```python
from build123d import *

# Parameters (mm, degrees)
F0_R     = 40
F1_DEPTH = 2.74
F2_R     = 8
F3_DEPTH = 40
F4_R     = 3.5
F5_DEPTH = 9.9
F7_DEPTH = 155.2


with BuildPart() as f1:
    # F0 (on Top) → F1 (new body)
    with BuildSketch(Plane.XY):
        Circle(F0_R)
    extrude(amount=F1_DEPTH)

    # F2 (on face) → F3 (join)
    with BuildSketch(Plane(origin=(0, 0, 0), x_dir=(1, 0, 0), z_dir=(0, 0, -1))):
        Circle(F2_R)
    extrude(amount=-F3_DEPTH)

    # F4 (on face) → F5 (join)
    with BuildSketch(Plane(origin=(0, 0, 0), x_dir=(1, 0, 0), z_dir=(0, 0, -1))):
        with BuildLine():
            Line((-38.7, -44.7), (38.7, -44.7))
            ThreePointArc((38.7, -44.7), (42.942641, -42.942641), (44.7, -38.7))
            Line((44.7, -38.7), (44.7, 38.7))
            ThreePointArc((44.7, 38.7), (42.942641, 42.942641), (38.7, 44.7))
            Line((38.7, 44.7), (-38.7, 44.7))
            ThreePointArc((-38.7, 44.7), (-42.942641, 42.942641), (-44.7, 38.7))
            Line((-44.7, 38.7), (-44.7, -38.7))
            ThreePointArc((-44.7, -38.7), (-42.942641, -42.942641), (-38.7, -44.7))
        make_face()
        with Locations((-35.355339, -35.355339)):
            Circle(F4_R, mode=Mode.SUBTRACT)
        with Locations((35.355339, -35.355339)):
            Circle(F4_R, mode=Mode.SUBTRACT)
        with Locations((-35.355339, 35.355339)):
            Circle(F4_R, mode=Mode.SUBTRACT)
        with Locations((35.355339, 35.355339)):
            Circle(F4_R, mode=Mode.SUBTRACT)
    extrude(amount=F5_DEPTH)

    # F6 (on face) → F7 (join)
    with BuildSketch(Plane(origin=(0, 0, -9.9), x_dir=(1, 0, 0), z_dir=(0, 0, -1))):
        with BuildLine():
            Line((44.7, 0), (44.7, 25.65))
            Line((44.7, 25.65), (31.65, 25.65))
            ThreePointArc((31.65, 25.65), (27.407359, 27.407359), (25.65, 31.65))
            Line((25.65, 31.65), (25.65, 44.7))
            Line((25.65, 44.7), (0, 44.7))
            Line((0, 44.7), (0, 0))
            Line((0, 0), (44.7, 0))
        make_face()
        with BuildLine():
            Line((44.7, -25.65), (44.7, 0))
            Line((44.7, 0), (0, 0))
            Line((0, 0), (0, -44.7))
            Line((0, -44.7), (25.65, -44.7))
            Line((25.65, -44.7), (25.65, -31.65))
            ThreePointArc((25.65, -31.65), (27.407359, -27.407359), (31.65, -25.65))
            Line((31.65, -25.65), (44.7, -25.65))
        make_face()
        with BuildLine():
            Line((-44.7, 0), (0, 0))
            Line((0, 0), (0, 44.7))
            Line((0, 44.7), (-25.65, 44.7))
            Line((-25.65, 44.7), (-25.65, 31.65))
            ThreePointArc((-25.65, 31.65), (-27.407359, 27.407359), (-31.65, 25.65))
            Line((-31.65, 25.65), (-44.7, 25.65))
            Line((-44.7, 25.65), (-44.7, 0))
        make_face()
        with BuildLine():
            Line((0, -44.7), (0, 0))
            Line((0, 0), (-44.7, 0))
            Line((-44.7, 0), (-44.7, -25.65))
            Line((-44.7, -25.65), (-31.65, -25.65))
            ThreePointArc((-31.65, -25.65), (-27.407359, -27.407359), (-25.65, -31.65))
            Line((-25.65, -31.65), (-25.65, -44.7))
            Line((-25.65, -44.7), (0, -44.7))
        make_face()
    extrude(amount=F7_DEPTH)


solid = f1.part
```
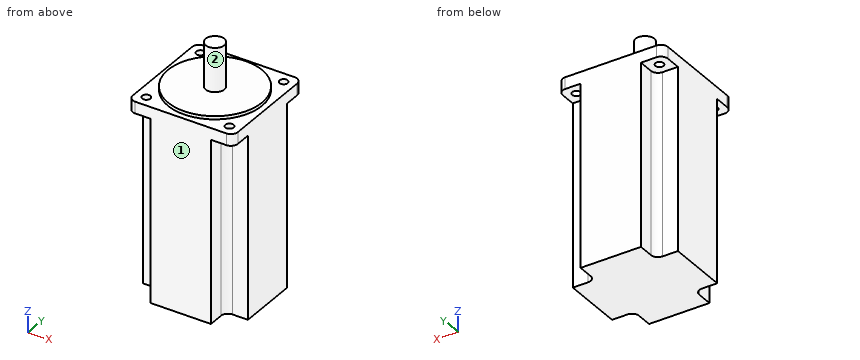
Part model, mm, in its own coordinate system. Face numbers are marked on the shaded views. A direction names the side the tool comes from. Give positions to 0.01 mm unless a question says otherwise; leave off trailing zeros. Order: outer loops, then holes, each group sorted by start corner. A loop starts at its lowest first (then second) coordinate and runs counter-clockwise, first axis right, second up. Notation, with made-up numbers: M -22,-39.75 L 8,-39.75 A14 cw 8,-28.75 Z; hole C 33.25,-36 d7. An arc over 180 degrees is marked long. Use a Markdown table: item, result. Add a question column.
(1) Saw through at B-B, the plane z = -123. Give the cut face in (x, y).
(2) Probe line 1 along Y through (x, z) = (-33, -6.5); line 2 along Z through (x, y) = (5, -15); line 3 along Z through (x, y) = (-41, 17). List the from-to ranges inside material, lowest first. Write a range as [from, to].
(3) 3-axis set-ups, long thin cutter, end or side, ignore diameter. For the marked faces 1 and 2: which of +Z, -Z, +X, -X, +Y, -Y reach the whole face in a straight line?
(4) Saw through at D-D, the plane x = -36. Give the cut face in (y, z), and give its area (3 significant figures).
(5) Drop flat-ended pins along their axis: P1, Ø14.5, axis at y = -41.5, z = -125, coming from the +X side; P2, Ø5.5, axis at x = -35.5, y = 39.5, coming from the -Z side; P3, Ø5, axis at y = -31, z = -132.5, coming from the +X side; P4, Ø4, axis at x = -35.36, y = -35.36, coming from the -Z side. Give the stop position or say it passes through.
(6) Saw through at A-A, the plane x = 0. Give the cut face in (y, z), and give its area (3 significant figures).
Answer key:
| question | item | result |
|---|---|---|
| 1 | outline | M -44.7,-25.65 L -31.65,-25.65 A6 cw -25.65,-31.65 L -25.65,-44.7 L 25.65,-44.7 L 25.65,-31.65 A6 cw 31.65,-25.65 L 44.7,-25.65 L 44.7,25.65 L 31.65,25.65 A6 cw 25.65,31.65 L 25.65,44.7 L -25.65,44.7 L -25.65,31.65 A6 cw -31.65,25.65 L -44.7,25.65 Z |
| 2 | line 1 | [-44.7, -37.94], [-32.77, 32.77], [37.94, 44.7] |
| 2 | line 2 | [-165.1, 2.74] |
| 2 | line 3 | [-165.1, 0] |
| 3 | face 1 | +Z, -Z, +X, -X, -Y |
| 3 | face 2 | +Z |
| 4 | outline | M -44.7,-9.9 L -38.8,-9.9 L -38.8,0 L -44.7,0 Z; M -31.92,-9.9 L -25.65,-9.9 L -25.65,-165.1 L 25.65,-165.1 L 25.65,-9.9 L 31.92,-9.9 L 31.92,0 L 17.44,0 L 17.44,2.74 L -17.44,2.74 L -17.44,0 L -31.92,0 Z; M 38.8,-9.9 L 44.7,-9.9 L 44.7,0 L 38.8,0 Z |
| 4 | area | 8,810 mm^2 |
| 5 | P1 | x = 25.65 |
| 5 | P2 | z = -9.9 |
| 5 | P3 | x = 26.54 |
| 5 | P4 | through |
| 6 | outline | M -44.7,-165.1 L 44.7,-165.1 L 44.7,0 L 40,0 L 40,2.74 L 8,2.74 L 8,40 L -8,40 L -8,2.74 L -40,2.74 L -40,0 L -44.7,0 Z |
| 6 | area | 15,600 mm^2 |
